Part model, mm, in its own coordinate system. A direction names the side the tool comes from. Give positions to 0.01 mm unless a question says otherwise; leave off trailing zeros. Order: outer loops, then holes, each group sorted by start corner. A loop starts at its lowest first (then second) coordinate and runs counter-clockwise, first axis right, second up. Notation, with made-up numbers: (-27, 77.25) -> (21, 77.25) arc R17 cw to (21, 88.25) -> close; hole circle Ø3 at (25, 79.25). An arc over 180 degrees is marked (long way). Write item = value, one per line. Start each with the question number.
Item 1: Flat gauge pins, fed straight in: P1, Ø4, axis at x = 6.5, y = 10.5, coming from the -Z side; P2, Ø1.5, axis at x = 25, y = 4.5, coming from the -Z side; P3, Ø2.5, axis at x = 29.5, y = -37.5, coming from the -Z side; P4, Ø4, axis at y = 33, z = 15.5, coming from the -X side (1 decimal). Where does each tip first touch, or does it go through?
Item 2: Band-saw the part on D-D on y = 12.5. Write the cut outline in (x, z), plus the area to 3 significant figures.
Item 3: Tool access for faces 4 (the face through (30, -38, 2.5)), 5 (the face through (29.362, 16.812, 13.823)), 6 (the face through (29.33, 40.67, 5.93)), 7 (the face through (30.1, -0.5, 12.8)): list every direction of +Z, -Z, +X, -X, +Y, -Y with a clear straight run to the whole face (end or side of a thin tool).
Item 4: Band-saw the part on C-C on y = 1. Write the cut outline in (x, z).
Item 5: Band-saw the part on B-B on x = 49. Write the cut outline in (y, z).
Item 6: Drill centre lines: line 1 along X through (y, z) = (-25, 17.5); line 2 along Y through (x, z) = (43, 1); line 3 along X through (y, z) = (-34.5, 29). Where is each one in solid material? Low to high.
Item 7: Pull direction X, two halves, no side cores. Call faces 1 (the face through (29.362, -1.136, 15.526)), 2 (the face through (2, -32, -2.5)), 3 (the face through (0, -9, 11)): +X half, -X half, draft (parallel to the pull), parting line (faces both ways), or undercut.
Item 8: Band-saw the part on A-A on z = 13.5. Write the cut outline in (x, y).
```python
from build123d import *

# Parameters (mm, degrees)
SKETCH3_W              = 79.5
SKETCH3_H              = 5
BOSS_EXTRUDE1_DEPTH    = 59.5
SKETCH4_W              = 55.5
SKETCH4_H              = 3
CUT_EXTRUDE1_DEPTH     = 80
SKETCH5_W              = 45.5
SKETCH5_H              = 2
CUT_EXTRUDE2_DEPTH     = 50
CUT_EXTRUDE3_START     = -3
CUT_EXTRUDE3_DEPTH     = 53.5
CUT_EXTRUDE4_START     = -5
CUT_EXTRUDE4_OUTLINE_W = 20
CUT_EXTRUDE4_OUTLINE_H = 3
CUT_EXTRUDE4_DEPTH     = 5


# Read off the part's stored shape, not the designer's step: Cut-Extrude4
with BuildPart() as part:
    # Sketch3 → Boss-Extrude1 (new body)
    with BuildSketch(Plane.YZ):
        Rectangle(SKETCH3_W, SKETCH3_H)
        Polygon((-39.75, 2.5), (39.75, 2.5), (-39.75, 23.801960798), align=None)
        Polygon((-39.75, 23.801960798), (-37.938266684, 30.563441582), (41.561733316, 9.261480784), (39.75, 2.5), align=None)
    extrude(amount=BOSS_EXTRUDE1_DEPTH)

    # Sketch4 → Cut-Extrude1 (cut)
    with BuildSketch(Plane(origin=(0, -43.0377451, 11.531929044), x_dir=(1, 0, 0), z_dir=(0, -0.9659258262890679, 0.25881904510252235))):
        with Locations((29.75, 16.202871609)):
            Rectangle(SKETCH4_W, SKETCH4_H)
    extrude(amount=-CUT_EXTRUDE1_DEPTH, mode=Mode.SUBTRACT)

    # Sketch5 → Cut-Extrude2 (cut)
    with BuildSketch(Plane(origin=(0, -43.0377451, 11.531929044), x_dir=(1, 0, 0), z_dir=(0, -0.9659258262890679, 0.25881904510252235))):
        with Locations((29.75, 18.702871609)):
            Rectangle(SKETCH5_W, SKETCH5_H)
    extrude(amount=-CUT_EXTRUDE2_DEPTH, mode=Mode.SUBTRACT)

    # Sketch6 → Cut-Extrude3 (cut)
    with BuildSketch(Plane.YZ.offset(59.5).offset(CUT_EXTRUDE3_START)):
        Polygon((-36.75, -6.898480781), (-36.75, 22.511144618), (36.75, 2.816878974), (36.75, -6.898480781), align=None)
    extrude(amount=-CUT_EXTRUDE3_DEPTH, mode=Mode.SUBTRACT)

    # Cut-Extrude4 outline → Cut-Extrude4 (cut)
    with BuildSketch(Plane(origin=(0, 0, -2.5), x_dir=(1, 0, 0), z_dir=(0, 0, -1)).offset(CUT_EXTRUDE4_START)):
        Polygon((56.5, 16.887495374), (56.5, -16.887495374), (59.5, -15.155444566), (59.5, 15.155444566), align=None)
        with Locations((29.75, -38.25)):
            Rectangle(CUT_EXTRUDE4_OUTLINE_W, CUT_EXTRUDE4_OUTLINE_H)
        with Locations((29.75, 38.25)):
            Rectangle(CUT_EXTRUDE4_OUTLINE_W, CUT_EXTRUDE4_OUTLINE_H)
        Polygon((0, -15.155444566), (3, -16.887495374), (3, 16.887495374), (0, 15.155444566), align=None)
    extrude(amount=CUT_EXTRUDE4_DEPTH, mode=Mode.SUBTRACT)


solid = part.part
```
Values found:
q1.P1 = 9.31
q1.P2 = 11.26
q1.P3 = 2.5
q1.P4 = through
q2.outline = (0, 2.5) -> (3, 2.5) -> (3, 9.31) -> (56.5, 9.31) -> (56.5, 2.5) -> (59.5, 2.5) -> (59.5, 17.05) -> (0, 17.05) -> close; hole (2, 11.87) -> (57.5, 11.87) -> (57.5, 14.98) -> (2, 14.98) -> close
q2.area = 329 mm^2
q3.face_4 = -Z, +Y, -Y
q3.face_5 = none
q3.face_6 = -Z, +X, -X, +Y
q3.face_7 = -Z
q4.outline = (0, 2.5) -> (3, 2.5) -> (3, 12.4) -> (56.5, 12.4) -> (56.5, 2.5) -> (59.5, 2.5) -> (59.5, 20.13) -> (52.5, 20.13) -> (52.5, 18.06) -> (57.5, 18.06) -> (57.5, 14.95) -> (2, 14.95) -> (2, 18.06) -> (7, 18.06) -> (7, 20.13) -> (0, 20.13) -> close
q5.outline = (-39.75, -2.5) -> (-36.75, -2.5) -> (-36.75, 22.51) -> (36.75, 2.82) -> (36.75, -2.5) -> (39.75, -2.5) -> (39.75, 2.5) -> (41.56, 9.26) -> (10.36, 17.62) -> (9.84, 15.69) -> (38.82, 7.93) -> (38.04, 5.03) -> (-39.23, 25.73) -> (-39.75, 23.8) -> close
q6.line_1 = 0 to 3, 56.5 to 59.5
q6.line_2 = -39.75 to -36.75, 36.75 to 39.75
q6.line_3 = 0 to 7, 52.5 to 59.5
q7.face_1 = undercut
q7.face_2 = draft
q7.face_3 = -X half
q8.outline = (0, -39.75) -> (59.5, -39.75) -> (59.5, 25.74) -> (0, 25.74) -> close; hole (2, 6.42) -> (57.5, 6.42) -> (57.5, 18.02) -> (2, 18.02) -> close; hole (3, -36.75) -> (56.5, -36.75) -> (56.5, -3.12) -> (3, -3.12) -> close
